Check sheet for the drawn part. Datum: minimum x, y, z corner. Units: mm. Coordinates: 2 decimals unless noted, no trailing zeros. Loops run counter-clockwise (first coordinate to the right, second up) from the corner with the lowest first, then second, coordinate; pieces in that order, holes last. Notation, with made-up numbers: (36, 83) -> (79, 83) arc R33 ccw to (79, 117) -> close; hole circle Ø6 at (88.25, -23.5). An arc over 180 degrees is marked (long way). Use CSV: the item, a comma, the result in double quotes. Start each with the question number.
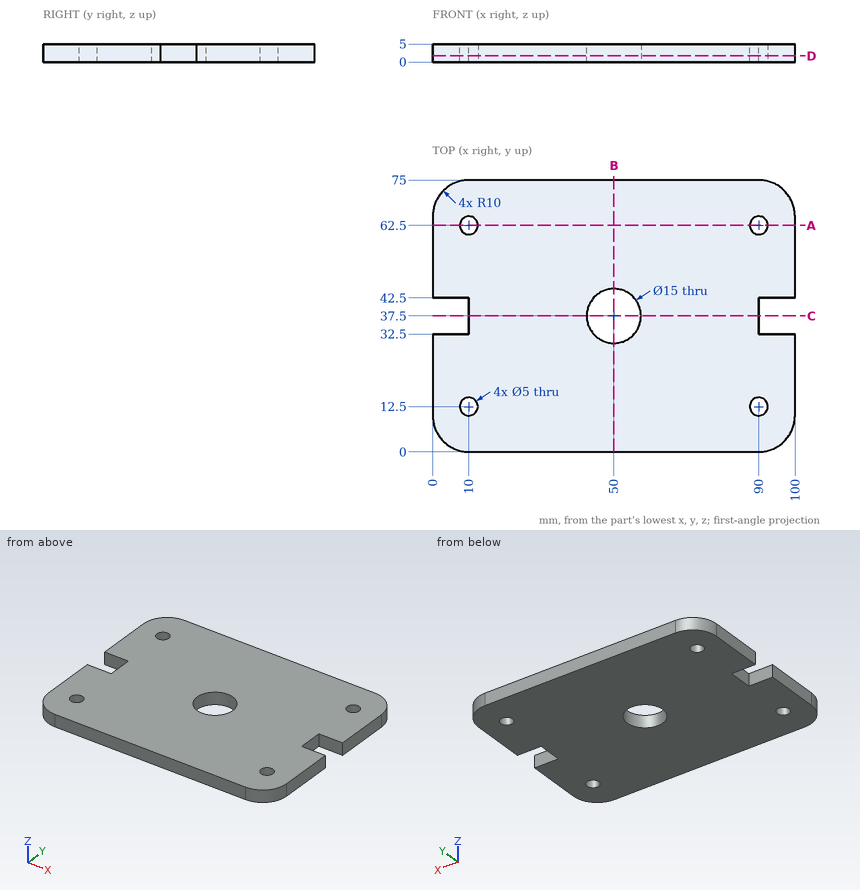
1. Cross-section at D-D, the plane z = 1.75. Record the boundary of the cut face in (x, y).
2. Cross-section at A-A, the plane y = 62.5. Record the boundary of the cut face in (x, z), plus the area to 3 significant figures.
3. Scan lines: line 1 (Y direction, x = 50, z = 3.8); line 2 (Y direction, x = 11, z = 2.95); line 3 (X direction, y = 37, z = 4.65). Record each from-to range of solid material in increasing order.
4. Cross-section at B-B, the plane x = 50. Record the boundary of the cut face in (y, z).
5. Depth check by flat-ended pin: pin 1 (1.5 mm diameter, centred on y = 37, z = 1.5, fed in from -X). Enter the tip coordinate at first touch or a pass-through.
6. Cross-section at C-C, the plane y = 37.5. Record the boundary of the cut face in (x, z).
Solution:
1,outline,"(0, 10) arc R10 ccw to (10, 0) -> (90, 0) arc R10 ccw to (100, 10) -> (100, 32.5) -> (90, 32.5) -> (90, 42.5) -> (100, 42.5) -> (100, 65) arc R10 ccw to (90, 75) -> (10, 75) arc R10 ccw to (0, 65) -> (0, 42.5) -> (10, 42.5) -> (10, 32.5) -> (0, 32.5) -> close; hole circle Ø5 at (10, 12.5); hole circle Ø5 at (10, 62.5); hole circle Ø15 at (50, 37.5); hole circle Ø5 at (90, 12.5); hole circle Ø5 at (90, 62.5)"
2,outline,"(0, 0) -> (7.5, 0) -> (7.5, 5) -> (0, 5) -> close; (12.5, 0) -> (87.5, 0) -> (87.5, 5) -> (12.5, 5) -> close; (92.5, 0) -> (100, 0) -> (100, 5) -> (92.5, 5) -> close"
2,area,"450 mm2"
3,line 1,"y = 0 to 30, 45 to 75"
3,line 2,"y = 0 to 10.21, 14.79 to 60.21, 64.79 to 75"
3,line 3,"x = 10 to 42.52, 57.48 to 90"
4,outline,"(0, 0) -> (30, 0) -> (30, 5) -> (0, 5) -> close; (45, 0) -> (75, 0) -> (75, 5) -> (45, 5) -> close"
5,pin 1,"stops at x = 10"
6,outline,"(10, 0) -> (42.5, 0) -> (42.5, 5) -> (10, 5) -> close; (57.5, 0) -> (90, 0) -> (90, 5) -> (57.5, 5) -> close"
